For this review, use the dimensioned drawing (mm, ordinates from the lowest corner) and the shaded views. Give positions to 0.01 mm unless a question says otherwise; leave off trailing zeros. Loops run counter-clockwise (first coordinate to the right, second up) from the corner with the lowest first, then second, coordinate; pieces in that order, holes last. Notation, with made-up numbers: M 57.5,13.5 L 72.5,13.5 A33 ccw 72.5,52.5 Z; hole C 57.5,-23.75 d2. An arc over 180 degrees is marked long. Use a Markdown table: item, result. Add a question column.
(1) Add section A-A, the plane x = 84.5. Give the boundary of the cut face in (y, z).
(2) Add section B-B, the plane z = 33.5. Give the boundary of the cut face in (x, y), then the cut area to 3 significant figures.
(3) Draft analysis for pull direction X (two halves, no side actions). For the marked faces 1 and 2, state which applies: pulls with the +X half, pulls with the -X half, needs draft (parallel to the pull), parting line crosses it, or undercut.
(4) For probe 1 along Y at (x, z) = (100, 8.5); probe 2 along X at (y, z) = (9.5, 33); probe 3 along X at (y, z) = (1.75, 18), list the stretches that pass through material, from the lowest coordinate up.
(5) Insertion check: pin 1 Ø4 at (y, z) = (8, 28) entering from +X. The pin has a flat end and moves straight along its axis. Give the tip position at first contact, or say it passes through.
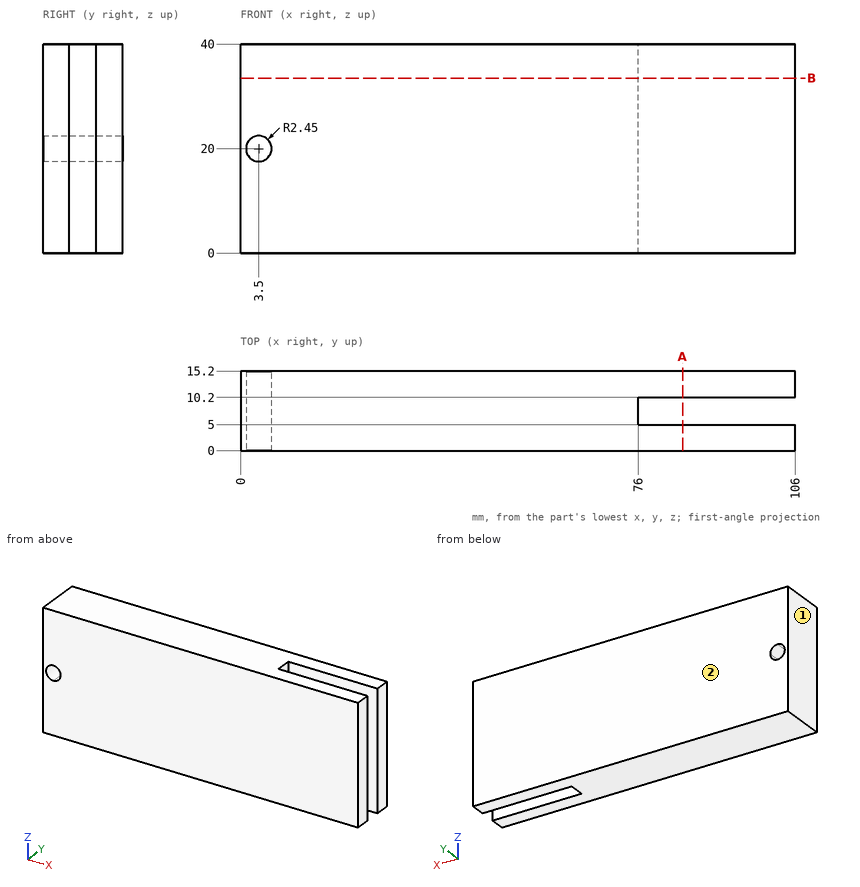
Established:
| question | item | result |
|---|---|---|
| 1 | outline | M 0,0 L 5,0 L 5,40 L 0,40 Z; M 10.2,0 L 15.2,0 L 15.2,40 L 10.2,40 Z |
| 2 | outline | M 0,0 L 106,0 L 106,5 L 76,5 L 76,10.2 L 106,10.2 L 106,15.2 L 0,15.2 Z |
| 2 | area | 1,460 mm^2 |
| 3 | face 1 | pulls with the -X half |
| 3 | face 2 | needs draft |
| 4 | probe 1 | 0 to 5, 10.2 to 15.2 |
| 4 | probe 2 | 0 to 76 |
| 4 | probe 3 | 0 to 2.08, 4.92 to 106 |
| 5 | pin 1 | x = 76 |
